from build123d import *

# Parameters (mm, degrees)
FLANGE_SKETCH_R      = 4
FLANGE_EXTRUDE_DEPTH = 0.5
JOINT_SKETCH_R       = 2.075
JOINT_EXTRUDE_DEPTH  = 6.3
HOLE_SKETCH_R        = 1
HOLE_EXTRUDE_DEPTH   = 10.235258524


with BuildPart() as part:
    # Flange Sketch → Flange Extrude (new, symmetric)
    with BuildSketch(Plane.XY):
        Circle(FLANGE_SKETCH_R)
    extrude(amount=FLANGE_EXTRUDE_DEPTH, both=True)

    # Joint Sketch → Joint Extrude (add)
    with BuildSketch(Plane.XY.offset(0.5)):
        Circle(JOINT_SKETCH_R)
    extrude(amount=JOINT_EXTRUDE_DEPTH)

    # Hole Sketch → Hole Extrude (cut, through all)
    with BuildSketch(Plane.XY.offset(6.8)):
        Circle(HOLE_SKETCH_R)
    extrude(amount=-HOLE_EXTRUDE_DEPTH, mode=Mode.SUBTRACT)


solid = part.part
Design review of the part built by this model. Coordinates are the model's own, in mm. Give positions to 0.01 mm unless a question says otherwise; leave off trailing zeros. Loops run counter-clockwise (first coordinate to the right, second up) from the corner with the lowest first, then second, coordinate; pieces in that order, holes last. Notation, with made-up numbers: (3.5, -13) - (52.5, -13) arc R29 cw to (52.5, 16) - close; hole circle Ø9 at (74, 66). An arc over 180 degrees is marked (long way). Use CSV: the item, a comma, the result in double quotes. Start each with the question number.
1. Wall thickness on L1, parallel to Y at x = 0, z = 1.5 (3 decimals); L2, parallel to Z at x = 3.25, y = -1.25; L3, parallel to Y at x = -1.5, z = 0.25: over which ranges is each line inside the solid? List them lowest first.
2. Add section C-C (z = 0.25). State the section outline as (x, y) points.
3. Add section A-A (x = 0). State the section outline as (y, z) points (3 decimals).
4. Add section D-D (x = 1.5). State the section outline as (y, z) points, plus the area to 3 significant figures.
5. Insertion check: P1, Ø2.5, axis at x = 0, y = 0, coming from the -Z side; P2, Ø3, axis at y = 1.5, z = 2.5, coming from the -X side (3 decimals); P3, Ø1, axis at x = 0.5, z = 3.5, coming from the +Y side (3 decimals); P4, Ø2, axis at x = -0.5, z = 5.5, coming from the -Y side (3 decimals). Each pin has a flat end and moves straight along its axis. Give the tip position at first contact, or say it passes through.
6. Draft analysis for pull direction X (two halves, no side actions). For faces 1 (the cylindrical face through (-0.45, -2.026, 3.606)), 2 (the cylindrical face through (0, -1, 3)), 3 (the flat face through (2, -2, 0.5)), state which applies: released by +X, released by -X, zero draft, split by the parting line, or undercut.
Results found:
1,L1,"y = -2.075 to -1, 1 to 2.075"
1,L2,"z = -0.5 to 0.5"
1,L3,"y = -3.71 to 3.71"
2,outline,"circle Ø8 at (0, 0); hole circle Ø2 at (0, 0)"
3,outline,"(-4, -0.5) - (-1, -0.5) - (-1, 6.8) - (-2.075, 6.8) - (-2.075, 0.5) - (-4, 0.5) - close; (1, -0.5) - (4, -0.5) - (4, 0.5) - (2.075, 0.5) - (2.075, 6.8) - (1, 6.8) - close"
4,outline,"(-3.71, -0.5) - (3.71, -0.5) - (3.71, 0.5) - (1.43, 0.5) - (1.43, 6.8) - (-1.43, 6.8) - (-1.43, 0.5) - (-3.71, 0.5) - close"
4,area,"25.5 mm²"
5,P1,"stops at z = -0.5"
5,P2,"stops at x = -2.075"
5,P3,"stops at y = 2.075"
5,P4,"stops at y = -2.075"
6,face 1,"split by the parting line"
6,face 2,"undercut"
6,face 3,"zero draft"
